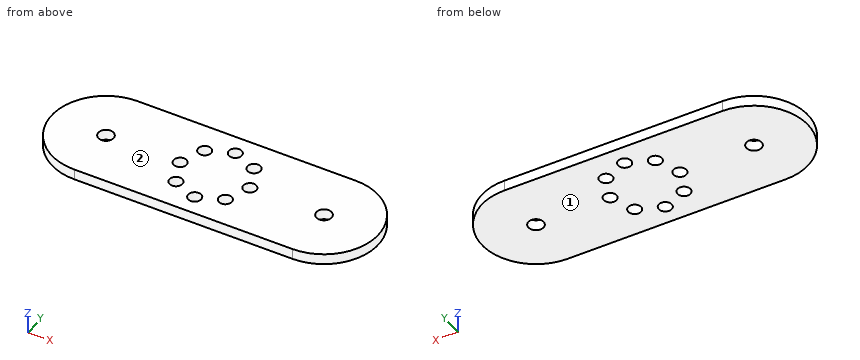
from build123d import *

# Parameters (mm, degrees)
SKETCH_1_R      = 3
SKETCH_1_R_2    = 3.5
EXTRUDE_1_DEPTH = 5


with BuildPart() as part:
    # 草图1 → 凸台-拉伸1 (new body)
    with BuildSketch(Plane.XY):
        with BuildLine():
            Line((-50, 25), (50, 25))
            ThreePointArc((50, 25), (75, 0), (50, -25))
            Line((50, -25), (-50, -25))
            ThreePointArc((-50, -25), (-75, 0), (-50, 25))
        make_face()
        with Locations((16, 0)):
            Circle(SKETCH_1_R, mode=Mode.SUBTRACT)
        with Locations((11.313708499, -11.313708499)):
            Circle(SKETCH_1_R, mode=Mode.SUBTRACT)
        with Locations((0, -16)):
            Circle(SKETCH_1_R, mode=Mode.SUBTRACT)
        with Locations((-11.313708499, -11.313708499)):
            Circle(SKETCH_1_R, mode=Mode.SUBTRACT)
        with Locations((-16, 0)):
            Circle(SKETCH_1_R, mode=Mode.SUBTRACT)
        with Locations((-11.313708499, 11.313708499)):
            Circle(SKETCH_1_R, mode=Mode.SUBTRACT)
        with Locations((0, 16)):
            Circle(SKETCH_1_R, mode=Mode.SUBTRACT)
        with Locations((11.313708499, 11.313708499)):
            Circle(SKETCH_1_R, mode=Mode.SUBTRACT)
        with Locations((-50, 0)):
            Circle(SKETCH_1_R_2, mode=Mode.SUBTRACT)
        with Locations((50, 0)):
            Circle(SKETCH_1_R_2, mode=Mode.SUBTRACT)
    extrude(amount=EXTRUDE_1_DEPTH)


solid = part.part
Part model, mm, in its own coordinate system. Face numbers are marked on the shaded views. Give positions to 0.01 mm unless a question says otherwise; leave off trailing zeros. Loops run counter-clockwise (first coordinate to the right, second up) from the corner with the lowest first, then second, coordinate; pieces in that order, holes last. Notation, with made-up numbers: M 43,-27.5 L 51,-27.5 A9 cw 51,-20.5 Z; hole C -19,-34 d1. An arc over 180 degrees is marked long. Put each result on its own line as item: value. Start each with the question number.
1) Probe probe 1 along Y at (x, z) = (50, 2.7); probe 2 along X at (y, z) = (11, 4.6); probe 3 along X at (y, z) = (-12.5, 1.4). List the from-to ranges inside material, lowest first.
2) Pull direction Z, two halves, no side cores. Call the marked faces 1 and 2: +Z half, -Z half, draft (parallel to the pull), parting line (faces both ways), or undercut.
3) Saw through at A-A (x = 0). List the corners of the cut face in (y, z).
4) Saw through at B-B (x = -16). List the corners of the cut face in (y, z), then the cut area to 3 significant figures.
5) Flat gauge pin, fed straight in: pin 1 (8 mm diameter, centred on x = 11.31, y = -11.31, fed in from -Z). Where does the tip first touch, or does it go through?
6) Saw through at C-C (y = -16). List the corners of the cut face in (x, z).
7) Saw through at D-D (z = 2.2). State how many separate pieces and enclosed holes the cut face has, then the cut area to 3 significant figures.
Numbers:
1. probe 1: -25 to -3.5, 3.5 to 25
1. probe 2: -72.45 to -14.3, -8.33 to 8.33, 14.3 to 72.45
1. probe 3: -71.65 to -14.07, -8.56 to 8.56, 14.07 to 71.65
2. face 1: -Z half
2. face 2: +Z half
3. outline: M -25,0 L -19,0 L -19,5 L -25,5 Z; M -13,0 L 13,0 L 13,5 L -13,5 Z; M 19,0 L 25,0 L 25,5 L 19,5 Z
4. outline: M -25,0 L -3,0 L -3,5 L -25,5 Z; M 3,0 L 25,0 L 25,5 L 3,5 Z
4. area: 220 mm^2
5. pin 1: z = 0
6. outline: M -69.21,0 L -3,0 L -3,5 L -69.21,5 Z; M 3,0 L 69.21,0 L 69.21,5 L 3,5 Z
7. separate pieces: 1
7. enclosed holes: 10
7. area: 6,660 mm^2
